CAD build for the part. Positions are in the model's coordinates, mm. Coordinates: 2 decimals unless noted, no trailing zeros. Write each loop counter-clockwise with the first axis right and the second up, starting at its lowest first coordinate (ties: lowest second). Pieces come first, ordered by that corner, then holes. Notation, with made-up numbers: (39.5, -15.75) - (46.5, -15.75) arc R18 ccw to (46.5, 2.25) - close; hole circle Ø11 at (48, -11.75). An arc over 180 degrees is marked (long way). One line per question, with ' | ' between items. Start each with the question number.
1. Band-saw the part on B-B, the plane z = 129.5. Write the cut outline in (x, y) (3 decimals).
2. Band-saw the part on C-C, the plane x = 8. Write the cut outline in (y, z) (3 decimals), then the cut area to 3 significant figures.
3. Probe line 1 (X direction, y = 0.8, z = 123.5) (3 decimals); line 2 (Z direction, x = 72, y = 0.3). List the from-to ranges inside material, lowest first.
4. Flat gauge pins, fed straight in: P1, Ø1, axis at x = 83.5, y = 2.5, coming from the -Z side; P2, Ø1.6, axis at y = 2, z = 127, coming from the -X side (3 decimals); P3, Ø1, axis at x = -112, y = 1.5, coming from the +Z side. Where does each tip first touch, or does it go through?
5. Band-saw the part on D-D, the plane z = 73. Write the cut outline in (x, y) (3 decimals).
6. Band-saw the part on A-A, the plane x = 58. Write the cut outline in (y, z) (3 decimals), then the cut area to 3 significant figures.
from build123d import *

# Parameters (mm, degrees)
BOSS_EXTRUDE1_DEPTH     = 3.175
CUT_EXTRUDE1_DEPTH      = 217.296510894
CUT_EXTRUDE1_DEPTH_BACK = 217.296510894
SKETCH3_W               = 60
SKETCH3_H               = 37
MIRROR1_DEPTH           = 3.175


# Read off the part's stored shape, not the designer's step: Mirror1
with BuildPart() as part:
    # Sketch1 → Boss-Extrude1 (new body)
    with BuildSketch(Plane(origin=(0, 0, 0), x_dir=(1, 0, 0), z_dir=(0, 1, 0))):
        Polygon((-139.7, 0), (0, 0), (0, 161.925), (-12.7, 161.925), (-12.7, 165.1), (-38.1, 165.1), (-38.1, 161.925), (-63.5, 161.925), (-63.5, 165.1), (-88.9, 165.1), (-88.9, 161.925), (-114.3, 161.925), (-114.3, 165.1), (-139.7, 165.1), (-139.7, 139.7), (-136.525, 139.7), (-136.525, 114.3), (-139.7, 114.3), (-139.7, 88.9), (-136.525, 88.9), (-136.525, 63.5), (-139.7, 63.5), (-139.7, 38.1), (-136.525, 38.1), (-136.525, 12.7), (-139.7, 12.7), align=None)
    extrude(amount=BOSS_EXTRUDE1_DEPTH)

    # Sketch3 → Cut-Extrude1 (cut, two sides: drawn at the far end of the back side and taken through both)
    with BuildSketch(Plane(origin=(0, 3.175, 0), x_dir=(1, 0, 0), z_dir=(0, 1, 0)).offset(-CUT_EXTRUDE1_DEPTH_BACK)):
        with Locations((-52.55, 132.4)):
            Rectangle(SKETCH3_W, SKETCH3_H)
        Polygon((-127, 165.1), (-127, 88.9), (-82.55, 88.9), (-82.55, 113.9), (-82.55, 150.9), (-82.55, 165.1), (-88.9, 165.1), (-88.9, 161.925), (-114.3, 161.925), (-114.3, 165.1), align=None)
    extrude(amount=CUT_EXTRUDE1_DEPTH + CUT_EXTRUDE1_DEPTH_BACK, mode=Mode.SUBTRACT)

    # Mirror1 outline → Mirror1 (add)
    with BuildSketch(Plane(origin=(0, 0, 0), x_dir=(1, 0, 0), z_dir=(0, 1, 0))):
        Polygon((139.7, 165.1), (127, 165.1), (127, 88.9), (82.55, 88.9), (82.55, 113.9), (22.55, 113.9), (22.55, 150.9), (82.55, 150.9), (82.55, 165.1), (63.5, 165.1), (63.5, 161.925), (38.1, 161.925), (38.1, 165.1), (12.7, 165.1), (12.7, 161.925), (0, 161.925), (0, 0), (-139.7, 0), (-139.7, -12.7), (-136.525, -12.7), (-136.525, -38.1), (-139.7, -38.1), (-139.7, -63.5), (-136.525, -63.5), (-136.525, -88.9), (-139.7, -88.9), (-139.7, -114.3), (-136.525, -114.3), (-136.525, -139.7), (-139.7, -139.7), (-139.7, -165.1), (-127, -165.1), (-127, -88.9), (-82.55, -88.9), (-82.55, -113.9), (-22.55, -113.9), (-22.55, -150.9), (-82.55, -150.9), (-82.55, -165.1), (-63.5, -165.1), (-63.5, -161.925), (-38.1, -161.925), (-38.1, -165.1), (-12.7, -165.1), (-12.7, -161.925), (12.7, -161.925), (12.7, -165.1), (38.1, -165.1), (38.1, -161.925), (63.5, -161.925), (63.5, -165.1), (82.55, -165.1), (82.55, -150.9), (22.55, -150.9), (22.55, -113.9), (82.55, -113.9), (82.55, -88.9), (127, -88.9), (127, -165.1), (139.7, -165.1), (139.7, -139.7), (136.525, -139.7), (136.525, -114.3), (139.7, -114.3), (139.7, -88.9), (136.525, -88.9), (136.525, -63.5), (139.7, -63.5), (139.7, -38.1), (136.525, -38.1), (136.525, -12.7), (139.7, -12.7), (139.7, 12.7), (136.525, 12.7), (136.525, 38.1), (139.7, 38.1), (139.7, 63.5), (136.525, 63.5), (136.525, 88.9), (139.7, 88.9), (139.7, 114.3), (136.525, 114.3), (136.525, 139.7), (139.7, 139.7), align=None)
    extrude(amount=MIRROR1_DEPTH)


solid = part.part
Filled in:
1) outline: (-136.525, 0) - (-127, 0) - (-127, 3.175) - (-136.525, 3.175) - close; (-22.55, 0) - (22.55, 0) - (22.55, 3.175) - (-22.55, 3.175) - close; (127, 0) - (136.525, 0) - (136.525, 3.175) - (127, 3.175) - close
2) outline: (0, -161.925) - (3.175, -161.925) - (3.175, 161.925) - (0, 161.925) - close | area: 1,030 mm²
3) line 1: x = -136.525 to -127, -22.55 to 22.55, 127 to 136.525 | line 2: z = -165.1 to -150.9, -113.9 to 113.9, 150.9 to 165.1
4) P1: stops at z = -88.9 | P2: stops at x = -136.525 | P3: stops at z = 88.9
5) outline: (-136.525, 0) - (136.525, 0) - (136.525, 3.175) - (-136.525, 3.175) - close
6) outline: (0, -161.925) - (3.175, -161.925) - (3.175, -150.9) - (0, -150.9) - close; (0, -113.9) - (3.175, -113.9) - (3.175, 113.9) - (0, 113.9) - close; (0, 150.9) - (3.175, 150.9) - (3.175, 161.925) - (0, 161.925) - close | area: 793 mm²
